Could you check a few things on this model? Use its own coordinates, in mm. Face numbers are marked on the shaded views. Coordinates: 2 decimals unless noted, no trailing zeros. Write each loop counter-clockwise with the first axis right and the second up, starting at its lowest first coordinate (ties: lowest second). Pieces come first, ordered by that corner, then holes. Notation, with made-up numbers: (42, -31.5) - (71, -31.5) arc R30 cw to (71, -7.5) - close; hole circle Ø3 at (24, 6). An arc over 180 degrees is marked (long way). Answer as a JSON object with one key per item and string values. Group by question number.
1) If we section it at A-A (y = 14): Write out the boundary of the cut face in (x, z).
2) Will these pins go through, and if not, where does the flat tip stop? pin 1 Ø12 at (x, z) = (-5, 17) entering from -Y; pin 2 Ø4 at (x, y) = (-21.5, 8.5) entering from +Z; pin 3 Ø4 at (y, z) = (16.5, 6) entering from +X.
3) Please list where these lines run through material, in increasing order: line 1 along Y through (x, z) = (-32.35, 0) (3 decimals); line 2 along X through (y, z) = (11, 6); line 3 along Y through (x, z) = (33, -1).
4) We'd pull the mould along Z, two halves only. Please class the marked faces 1 and 2: released by +Z, released by -Z, zero draft, split by the parting line, or undercut.
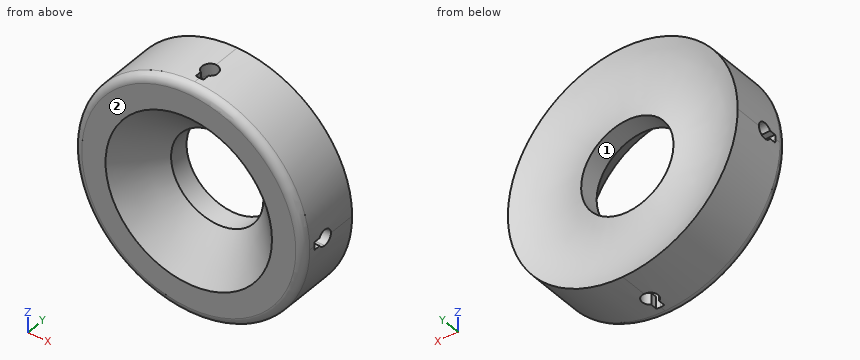
```python
from build123d import *
from build123d.topology import SkipClean

# Parameters (mm, degrees)
SKETCH1_R           = 36.83
BOSS_EXTRUDE1_DEPTH = 20.32
FILLET1_R           = 2.54
SKETCH2_R           = 26.67
SKETCH3_R           = 14.7955
SKETCH4_R           = 14.7955
CUT_EXTRUDE1_DEPTH  = 76.2
SKETCH8_R           = 2.54
CUT_EXTRUDE2_DEPTH  = 6.35
CIRPATTERN1_COUNT   = 4
CUT_EXTRUDE3_DEPTH  = 6.35
SKETCH10_R          = 4.445
CUT_EXTRUDE4_DEPTH  = 2.54
BOSS_EXTRUDE2_DEPTH = 2.54
BOSS_EXTRUDE3_DEPTH = 6.35
SKETCH13_R          = 39.975148753
SKETCH13_R_2        = 36.83
CUT_EXTRUDE5_DEPTH  = 21.59
CIRPATTERN2_COUNT   = 4


with BuildPart() as part:
    # Sketch1 → Boss-Extrude1 (new body)
    with BuildSketch(Plane(origin=(0, 0, 0), x_dir=(1, 0, 0), z_dir=(0, 1, 0))):
        with Locations(Location((0, 0, 0), (0, 0, 270))):
            Circle(SKETCH1_R)
    extrude(amount=BOSS_EXTRUDE1_DEPTH)

    # Fillet1
    fillet1_edges = [part.edges().sort_by_distance(p)[0] for p in [
        (0, 0, -36.83),
    ]]
    fillet(fillet1_edges, radius=FILLET1_R)

    # Sketch2 → Cut-Loft1 section 0
    with BuildSketch(Plane(origin=(0, 0, 0), x_dir=(1, 0, 0), z_dir=(0, 1, 0))):
        Circle(SKETCH2_R)
    # Sketch3 → Cut-Loft1 section 1
    with BuildSketch(Plane(origin=(0, 11.938, 0), x_dir=(1, 0, 0), z_dir=(0, 1, 0))):
        Circle(SKETCH3_R)
    loft(mode=Mode.SUBTRACT)

    # Sketch4 → Cut-Extrude1 (cut)
    with BuildSketch(Plane.XZ.offset(-11.938)):
        with Locations(Location((0, 0, 0), (0, 0, 270))):
            Circle(SKETCH4_R)
    extrude(amount=-CUT_EXTRUDE1_DEPTH, mode=Mode.SUBTRACT)

    # Sketch8 → Cut-Extrude2 (cut)
    with BuildSketch(Plane.XY.offset(36.83)):
        with Locations((0, 8.89)):
            Circle(SKETCH8_R)
    cut_extrude2 = extrude(amount=-CUT_EXTRUDE2_DEPTH, mode=Mode.SUBTRACT)

    # CirPattern1: Cut-Extrude2 ×4 about axis
    cirpattern1_axis = Axis((0, 0, 0), (0, 1, 0))
    for i in range(1, CIRPATTERN1_COUNT):
        add(cut_extrude2.rotate(cirpattern1_axis, i * 360 / CIRPATTERN1_COUNT), mode=Mode.SUBTRACT)

    # Sketch9 → Cut-Extrude3 (cut)
    with BuildSketch(Plane.XY.offset(36.83)):
        with BuildLine():
            Line((-1.27, 4.445), (1.27, 4.445))
            Line((1.27, 4.445), (1.27, 6.690295474))
            ThreePointArc((1.27, 6.690295474), (0, 6.35), (-1.27, 6.690295474))
            Line((-1.27, 6.690295474), (-1.27, 4.445))
        make_face()
    cut_extrude3 = extrude(amount=-CUT_EXTRUDE3_DEPTH, mode=Mode.SUBTRACT)

    # Sketch10 → Cut-Extrude4 (cut)
    with BuildSketch(Plane.XY.offset(30.48)):
        with Locations((0, 8.89)):
            Circle(SKETCH10_R)
    cut_extrude4 = extrude(amount=CUT_EXTRUDE4_DEPTH, mode=Mode.SUBTRACT)

    # Sketch11 → Boss-Extrude2 (add)
    with BuildSketch(Plane.XY.offset(30.48)):
        with BuildLine():
            Line((-2.54, 8.89), (-4.445, 8.89))
            ThreePointArc((-4.445, 8.89), (2.656395584, 12.453928661), (1.27, 4.630290503))
            Line((1.27, 4.630290503), (1.27, 6.690295474))
            ThreePointArc((1.27, 6.690295474), (1.27, 11.089704526), (-2.54, 8.89))
        make_face()
    boss_extrude2 = extrude(amount=BOSS_EXTRUDE2_DEPTH)

    # Sketch12 → Boss-Extrude3 (add)
    with BuildSketch(Plane.XY.offset(30.48)):
        with BuildLine():
            Line((-1.27, 4.445), (-1.1e-08, 4.445))
            ThreePointArc((-1.1e-08, 4.445), (-0.641722798, 4.491566546), (-1.27, 4.630290503))
            Line((-1.27, 4.630290503), (-1.27, 4.445))
        make_face()
        with BuildLine():
            Line((-1.1e-08, 4.445), (1.27, 4.445))
            Line((1.27, 4.445), (1.27, 4.630290503))
            ThreePointArc((1.27, 4.630290503), (0.641722787, 4.491566544), (-1.1e-08, 4.445))
        make_face()
    boss_extrude3 = extrude(amount=BOSS_EXTRUDE3_DEPTH)

    # Sketch13 → Cut-Extrude5 (cut)
    with BuildSketch(Plane.XZ):
        Circle(SKETCH13_R)
        with Locations(Location((0, 0, 0), (0, 0, 90))):
            Circle(SKETCH13_R_2, mode=Mode.SUBTRACT)
    cut_extrude5 = extrude(amount=-CUT_EXTRUDE5_DEPTH, mode=Mode.SUBTRACT)

    # CirPattern2: Cut-Extrude3, Cut-Extrude4, Boss-Extrude2, Boss-Extrude3, Cut-Extrude5 ×4 about axis
    with SkipClean():  # the faces are left unmerged after this step: merging them gives an invalid solid
        cirpattern2_axis = Axis((0, 0, 0), (0, 1, 0))
        add([cut_extrude3.rotate(cirpattern2_axis, i * 360 / CIRPATTERN2_COUNT) for i in range(1, CIRPATTERN2_COUNT)], mode=Mode.SUBTRACT)
        add([cut_extrude4.rotate(cirpattern2_axis, i * 360 / CIRPATTERN2_COUNT) for i in range(1, CIRPATTERN2_COUNT)], mode=Mode.SUBTRACT)
        add([boss_extrude2.rotate(cirpattern2_axis, i * 360 / CIRPATTERN2_COUNT) for i in range(1, CIRPATTERN2_COUNT)])
        add([boss_extrude3.rotate(cirpattern2_axis, i * 360 / CIRPATTERN2_COUNT) for i in range(1, CIRPATTERN2_COUNT)])
        add([cut_extrude5.rotate(cirpattern2_axis, i * 360 / CIRPATTERN2_COUNT) for i in range(1, CIRPATTERN2_COUNT)], mode=Mode.SUBTRACT)
    add(part.part.scale(1), mode=Mode.REPLACE)  # the faces are merged on a copy

    # Sketch17 → Cut-Revolve1 (revolve, cut)
    with BuildSketch(Plane(origin=(0, 0, 0), x_dir=(0, 0, -1), z_dir=(1, 0, 0))):
        with BuildLine():
            Line((36.83, 20.32), (14.7955, 20.32))
            Line((14.7955, 20.32), (14.7955, 18.415))
            ThreePointArc((14.7955, 18.415), (25.983986176, 17.386868237), (36.83, 20.32))
        make_face()
    revolve(axis=Axis((0, 0, 0), (0, 1, 0)), mode=Mode.SUBTRACT)


solid = part.part
```
Here are the results:
{
 "1": {"outline": "circle Ø73.66 at (0, 0); hole circle Ø29.59 at (0, 0)"},
 "2": {"pin 1": "stops at y = 2.97", "pin 2": "stops at z = 31.24", "pin 3": "stops at x = 36.61"},
 "3": {"line 1": "y = 0 to 4.445, 11.43 to 18.601", "line 2": "x = -36.34 to -14.54, 14.54 to 36.34", "line 3": "y = 0 to 4.56, 11.22 to 18.81"},
 "4": {"face 1": "undercut", "face 2": "zero draft"}
}
